Verification items for the finished model (mm, model axes). Give positions to 0.01 mm unless a question says otherwise; leave off trailing zeros. Loops run counter-clockwise (first coordinate to the right, second up) from the corner with the lowest first, then second, coordinate; pieces in that order, holes last. Notation, with made-up numbers: (-6, -28) -> (21, -28) arc R21 ccw to (21, -5) -> close; hole circle Ø5 at (34.25, -26). An arc over 180 degrees is marked (long way). Answer in a Markdown table with one row per item. Add a question column.
Q1. Release check for a two-part mould opening along X. For faces 1 (the face through (20.141, -3.131, -28.656)), 2 (the face through (-81.397, -3, 12)), 3 (the face through (-3, 0, 12)) record: pulls with the +X half, pulls with the -X half, needs draft (parallel to the pull), parting line crosses it, or undercut.
Q2. Material ranges on probe 1 along X at (y, z) = (-1.75, 39); probe 2 along Z at (x, y) = (28, -1.75); probe 3 along Z at (x, y) = (-63, -1), recorded low to high.
Q3. Section check C-C on x = -67.5. Enter the section's corners in (y, z), and give its area (3 significant figures).
Q4. Section check A-A on y = -1. Enter the section's corners in (x, z) (3 decimals), and give its area (3 significant figures).
Q5. Section check B-B on z = 38.1. Enter the section's corners in (x, y), and give its area (3 significant figures).
```python
from build123d import *

# Parameters (mm, degrees)
F0_R     = 9.525
F0_W     = 136.144
F0_H     = 30.48
F0_W_2   = 23.876
F1_DEPTH = 6.35


with BuildPart() as f1:
    # F0 (on Front) → F1 (new body)
    with BuildSketch(Plane.XZ):
        Polygon((78.622635, 91.990085), (-81.397365, 91.990085), (-81.397365, 15.24), (54.746635, 15.24), (78.622635, 15.24), align=None)
        with Locations((-67.981206, 38.1)):
            Circle(F0_R, mode=Mode.SUBTRACT)
        with Locations((20.918794, 38.1)):
            Circle(F0_R, mode=Mode.SUBTRACT)
        with Locations((-13.325365, 0)):
            Rectangle(F0_W, F0_H)
        with Locations((66.684635, 0)):
            Rectangle(F0_W_2, F0_H)
        Polygon((54.746635, -15.24), (-81.397365, -15.24), (-81.397365, -70.67487), (78.622635, -70.67487), (78.622635, -15.24), align=None)
        with Locations((-67.518748, -38.1)):
            Circle(F0_R, mode=Mode.SUBTRACT)
        with Locations((21.381252, -38.1)):
            Circle(F0_R, mode=Mode.SUBTRACT)
    extrude(amount=F1_DEPTH)


solid = f1.part
```
Taken from the geometry:
| question | item | result |
|---|---|---|
| 1 | face 1 | undercut |
| 1 | face 2 | pulls with the -X half |
| 1 | face 3 | needs draft |
| 2 | probe 1 | x = -81.4 to -77.46, -58.5 to 11.44, 30.4 to 78.62 |
| 2 | probe 2 | z = -70.67 to -44.95, -31.25 to 31.73, 44.47 to 91.99 |
| 2 | probe 3 | z = -70.67 to -46.48, -29.72 to 29.98, 46.22 to 91.99 |
| 3 | outline | (-6.35, -70.67) -> (0, -70.67) -> (0, -47.62) -> (-6.35, -47.62) -> close; (-6.35, -28.58) -> (0, -28.58) -> (0, 28.59) -> (-6.35, 28.59) -> close; (-6.35, 47.61) -> (0, 47.61) -> (0, 91.99) -> (-6.35, 91.99) -> close |
| 3 | area | 791 mm² |
| 4 | outline | (-81.397, -70.675) -> (78.623, -70.675) -> (78.623, 91.99) -> (-81.397, 91.99) -> close; hole circle Ø19.05 at (-67.981, 38.1); hole circle Ø19.05 at (-67.519, -38.1); hole circle Ø19.05 at (20.919, 38.1); hole circle Ø19.05 at (21.381, -38.1) |
| 4 | area | 24,900 mm² |
| 5 | outline | (-81.4, -6.35) -> (-77.51, -6.35) -> (-77.51, 0) -> (-81.4, 0) -> close; (-58.46, -6.35) -> (11.39, -6.35) -> (11.39, 0) -> (-58.46, 0) -> close; (30.44, -6.35) -> (78.62, -6.35) -> (78.62, 0) -> (30.44, 0) -> close |
| 5 | area | 774 mm² |
